Input: part model. Units: mm. Frame: model coordinates. Coordinates: 2 decimals unless noted, no trailing zeros. Order: outer loops, then holes, each group sorted by start corner. A loop starts at its lowest first (then second) coordinate and runs counter-clockwise, first axis right, second up. Notation, with made-up numbers: (18.25, 0) -> (66.25, 0) arc R25 ccw to (66.25, 29) -> close; hole circle Ø11 at (-8.5, 21). An arc over 180 degrees is marked (long way). One line per question, with ' | ' between items.
```python
from build123d import *

# Parameters (mm, degrees)
F0_W     = 762
F0_H     = 101.6
F0_R     = 12.7
F1_DEPTH = 6.35
F2_W     = 9.525
F2_H     = 50.8
F3_DEPTH = 25.4
F4_SIZE  = 12.7
F5_R     = 0.9144


with BuildPart() as f1:
    # F0 (on Front) → F1 (new body)
    with BuildSketch(Plane.XZ):
        with Locations((381, 50.8)):
            Rectangle(F0_W, F0_H)
        with Locations((63.5, 50.8)):
            Circle(F0_R, mode=Mode.SUBTRACT)
        with Locations((190.5, 50.8)):
            Circle(F0_R, mode=Mode.SUBTRACT)
        with Locations((317.5, 50.8)):
            Circle(F0_R, mode=Mode.SUBTRACT)
        with Locations((444.5, 50.8)):
            Circle(F0_R, mode=Mode.SUBTRACT)
        with Locations((571.5, 50.8)):
            Circle(F0_R, mode=Mode.SUBTRACT)
        with Locations((698.5, 50.8)):
            Circle(F0_R, mode=Mode.SUBTRACT)
    extrude(amount=F1_DEPTH)

    # F2 (on face) → F3 (cut)
    with BuildSketch(Plane.XZ.offset(6.35)):
        with Locations((98.4377, 50.8)):
            Rectangle(F2_W, F2_H)
        with Locations((111.1377, 50.8)):
            Rectangle(F2_W, F2_H)
        with Locations((123.8377, 50.8)):
            Rectangle(F2_W, F2_H)
        with Locations((136.5377, 50.8)):
            Rectangle(F2_W, F2_H)
        with Locations((149.2377, 50.8)):
            Rectangle(F2_W, F2_H)
        with Locations((225.4377, 50.8)):
            Rectangle(F2_W, F2_H)
        with Locations((238.1377, 50.8)):
            Rectangle(F2_W, F2_H)
        with Locations((250.8377, 50.8)):
            Rectangle(F2_W, F2_H)
        with Locations((263.5377, 50.8)):
            Rectangle(F2_W, F2_H)
        with Locations((276.2377, 50.8)):
            Rectangle(F2_W, F2_H)
        with Locations((352.4377, 50.8)):
            Rectangle(F2_W, F2_H)
        with Locations((365.1377, 50.8)):
            Rectangle(F2_W, F2_H)
        with Locations((377.8377, 50.8)):
            Rectangle(F2_W, F2_H)
        with Locations((390.5377, 50.8)):
            Rectangle(F2_W, F2_H)
        with Locations((403.2377, 50.8)):
            Rectangle(F2_W, F2_H)
        with Locations((479.4377, 50.8)):
            Rectangle(F2_W, F2_H)
        with Locations((492.1377, 50.8)):
            Rectangle(F2_W, F2_H)
        with Locations((504.8377, 50.8)):
            Rectangle(F2_W, F2_H)
        with Locations((517.5377, 50.8)):
            Rectangle(F2_W, F2_H)
        with Locations((530.2377, 50.8)):
            Rectangle(F2_W, F2_H)
        with Locations((606.4377, 50.8)):
            Rectangle(F2_W, F2_H)
        with Locations((619.1377, 50.8)):
            Rectangle(F2_W, F2_H)
        with Locations((631.8377, 50.8)):
            Rectangle(F2_W, F2_H)
        with Locations((644.5377, 50.8)):
            Rectangle(F2_W, F2_H)
        with Locations((657.2377, 50.8)):
            Rectangle(F2_W, F2_H)
    extrude(amount=-F3_DEPTH, mode=Mode.SUBTRACT)

    # F4
    f4_edges = [f1.edges().sort_by_distance(p)[0] for p in [
        (762, -3.175, 101.6),
        (762, -3.175, 0),
        (0, -3.175, 0),
        (0, -3.175, 101.6),
    ]]
    chamfer(f4_edges, length=F4_SIZE)

    # F5
    f5_edges = [f1.edges().sort_by_distance(p)[0] for p in [
        (6.35, -6.35, 95.25),
        (381, -6.35, 101.6),
        (0, 0, 50.8),
        (381, -6.35, 0),
        (6.35, -6.35, 6.35),
        (755.65, -6.35, 95.25),
        (755.65, -6.35, 6.35),
        (762, -6.35, 50.8),
        (381, 0, 101.6),
        (6.35, 0, 95.25),
        (0, -6.35, 50.8),
        (6.35, 0, 6.35),
        (381, 0, 0),
        (755.65, 0, 6.35),
        (762, 0, 50.8),
    ]]
    fillet(f5_edges, radius=F5_R)


solid = f1.part
```
1. Cut plane B-B, the plane z = 50.8. State how many separate pieces and enclosed holes the cut face has, and give its area (3 significant figures).
Recorded:
separate pieces: 32 | enclosed holes: 0 | area: 2,360 mm^2
2. Ray query, line 1 (Z direction, x = 698.5, y = -3.75); line 2 (Z direction, x = 387, y = -3.25); line 3 (X direction, y = -1.25, z = 9.5). Return the intervals inside material, ascending. Write a range as [from, to].
Recorded:
line 1: z = [0, 38.1], [63.5, 101.6] | line 2: z = [0, 25.4], [76.2, 101.6] | line 3: x = [3.2, 758.8]
3. Cut plane A-A, the plane x = 190.5. Return loops of the section in (y, z), and give its area (3 significant figures).
Recorded:
outline: (-6.35, 0.91) arc R0.91 ccw to (-5.44, 0) -> (-0.91, 0) arc R0.91 ccw to (0, 0.91) -> (0, 38.1) -> (-6.35, 38.1) -> close; (-6.35, 63.5) -> (0, 63.5) -> (0, 100.69) arc R0.91 ccw to (-0.91, 101.6) -> (-5.44, 101.6) arc R0.91 ccw to (-6.35, 100.69) -> close | area: 483 mm^2
4. Pin query (flat end, axial travel): pin 1 Ø2 at (x, z) = (458.5, 68) entering from +Y; pin 2 Ø15 at (x, z) = (317.5, 50.8) entering from +Y. Return the tip coordinate at first contact, or that it passes through.
Recorded:
pin 1: stops at y = 0 | pin 2: passes through
5. Mould query, pull axis X, two halves, no side actions, for faces 1 (the face through (685.812, -3.131, 51.358)), 2 (the face through (376, -6.35, 85)), 3 (the face through (6.63, -0.26, 6.46)). Classes: released by +X, released by -X, zero draft, split by the parting line, or undercut.
Recorded:
face 1: undercut | face 2: zero draft | face 3: released by -X
